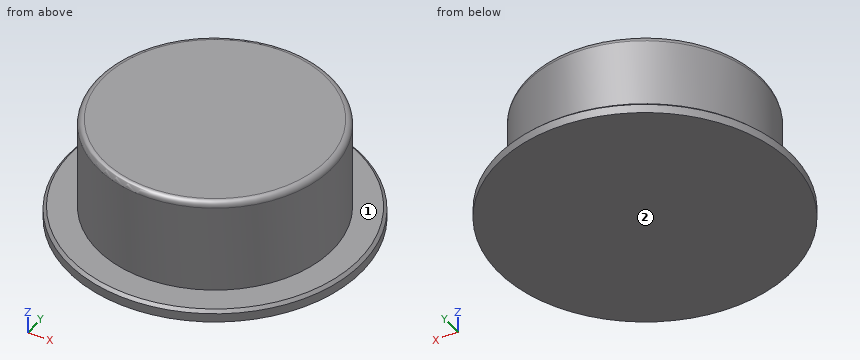
from build123d import *

# Parameters (mm, degrees)
CHANFREIN1_SIZE = 0.1


with BuildPart() as part:
    # Esquisse1 → Révolution1 (revolve)
    with BuildSketch(Plane.XZ, mode=Mode.PRIVATE) as r_volution1_sk:
        with BuildLine():
            Line((3.8, 3.6), (0, 3.6))
            Line((0, 3.6), (0, 0))
            Line((0, 0), (5, 0))
            Line((5, 0), (5, 0.4))
            Line((5, 0.4), (4, 0.4))
            Line((4, 0.4), (4, 3.4))
            ThreePointArc((4, 3.4), (3.941421356, 3.541421356), (3.8, 3.6))
        make_face()
    revolve(r_volution1_sk.sketch.rotate(Axis((0, 0, 3.6), (0, 0, -1)), 180), axis=Axis((0, 0, 3.6), (0, 0, -1)))

    # Chanfrein1
    chanfrein1_edges = [part.edges().sort_by_distance(p)[0] for p in [
        (5, 0, 0.4),
    ]]
    chamfer(chanfrein1_edges, length=CHANFREIN1_SIZE)


solid = part.part
Can you work these out from the model? Positions are in its coordinate system, mm. Face numbers are marked on the shaded views. A direction names the side the tool comes from. Round coordinates to 2 decimals unless told otherwise and drop trailing zeros. Order: outer loops, then holes, each group sorted by start corner. A loop starts at its lowest first (then second) coordinate and runs counter-clockwise, first axis right, second up. Notation, with made-up numbers: (-20, 78.25) - (18, 78.25) arc R16 cw to (18, 94.25) - close; hole circle Ø5 at (69, 34.25). An arc over 180 degrees is marked (long way). Answer in a Markdown table with one row per item.
(1) Which directions (+Z, -Z, +X, -X, +Y, -Y) give clear straight access to the entire face, cutting with the end or side of a thin tool? Please do the marked faces 1 and 2.
From the geometry:
| item | result |
|---|---|
| face 1 | +Z |
| face 2 | -Z, +X, -X, +Y, -Y |
(2) Suppose I cut it at A-A, the plane x = 0. Please give me the cut outline in (y, z).
From the geometry:
| item | result |
|---|---|
| outline | (-5, 0) - (5, 0) - (5, 0.3) - (4.9, 0.4) - (4, 0.4) - (4, 3.4) arc R0.2 ccw to (3.8, 3.6) - (-3.8, 3.6) arc R0.2 ccw to (-4, 3.4) - (-4, 0.4) - (-4.9, 0.4) - (-5, 0.3) - close |
(3) Please list where these lines run through material, in increasing order: L1, parallel to Z at x = 2.75, y = -3.5; L2, parallel to Z at x = 0.75, y = -3.75; L3, parallel to Y at x = -1, z = 0.35. Write a range as from..to.
From the geometry:
| item | result |
|---|---|
| L1 | z = 0..0.4 |
| L2 | z = 0..3.6 |
| L3 | y = -4.85..4.85 |
(4) For P1, Ø1.5, axis at x = 0.5, z = 1.5, coming from the +Y side, with a flat end and sliding along its axis, tell me the tip position at first contact or that it passes through.
From the geometry:
| item | result |
|---|---|
| P1 | stops at y = 4 |
(5) Suppose I cut it at C-C, the plane z = 1.15. Please give me the cut outline in (x, y).
From the geometry:
| item | result |
|---|---|
| outline | circle Ø8 at (0, 0) |
